For this review, take the finished solid that the model builds, in its own axes (mm). Face numbers are marked on the shaded views. A direction names the side the tool comes from. Coordinates: 2 decimals unless noted, no trailing zeros. Loops run counter-clockwise (first coordinate to the right, second up) from the corner with the lowest first, then second, coordinate; pieces in that order, holes last.
1. Mouldability with a two-part tool opening along X and no side actions: class the marked faces 1, 2, 3 and 4 as pulls with the +X half, pulls with the -X half, needs draft (parallel to the pull), parting line crosses it, or undercut.
2. Clearance check with flat-ended pins moving along their axes: P1, Ø3, axis at x = -59, z = 13, coming from the -Y side; P2, Ø1.5, axis at y = 9.5, z = 23, coming from the -X side; P3, Ø1, axis at x = -65.5, y = 8, coming from the -Z side. State where each tip first meets the part, or that it passes through.
3. Take a section at A-A, the plane x = 23.5. State the section outline as (y, z) points (3 decimals).
4. Machinability: for the marked faces 5 and 6, which of the approach directions +Z, -Z, +X, -X, +Y, -Y give a long, thin tool a straight path to every point of the face, cutting with its end or side? Answer none if there is none.
5. Take a section at B-B, the plane y = -9.5. State the section outline as (x, z) points.
6. To check wall thickness, follow probe 1 along Y at (x, z) = (-24.5, 4.5) (3 decimals); probe 2 along Z at (x, y) = (45.5, 2.5); probe 3 along X at (y, z) = (5, 9). State the ranges of each line that lie inside material, in increasing order.
```python
from build123d import *

# Parameters (mm, degrees)
F0_W        = 177.8
F0_H        = 44.45
F1_DEPTH    = 31.75
F2_W        = 2.032
F2_H        = 5.08
F2_H_2      = 2.957622528
F3_DEPTH    = 70.866
F4_T1_DEPTH = 472.3767319638
F5_R        = 10.16
F6_R        = 10.16
F7_R        = 8.5849434278
F8_W        = 78.1799629331
F8_H        = 27.9869418591
F9_DEPTH    = 12.7


# Not quite as in the source:
# - a fillet or chamfer that OpenCascade refuses, or shapes differently, is made with other operations: its cross-section is extruded or revolved along the edge and cut away or added


with BuildPart() as f1:
    # F0 (on Top) → F1 (new body)
    with BuildSketch(Plane.XY):
        Rectangle(F0_W, F0_H)
    extrude(amount=F1_DEPTH)

    # F2 (on Front) → F3 (cut, symmetric)
    with BuildSketch(Plane.XZ):
        with Locations((-65.8876, 0)):
            Rectangle(F2_W, F2_H)
        with Locations((45.8724, 1.061188736)):
            Rectangle(F2_W, F2_H_2)
    extrude(amount=F3_DEPTH, both=True, mode=Mode.SUBTRACT)

    # F4: fillet of radius 131.2269923964 on 1 edges, made by hand

    # F4_s2 → F4_t1 (cut)
    with BuildSketch(Plane.XZ.offset(-236.1883659819)):
        with BuildLine():
            ThreePointArc((-3.3146536072, 31.75), (-48.9570517069, 23.5567226134), (-88.9, 0))
            Line((-88.9, 0), (-88.9, 31.75))
            Line((-88.9, 31.75), (-3.3146536072, 31.75))
        make_face()
    extrude(amount=F4_T1_DEPTH, mode=Mode.SUBTRACT)

    # F5
    f5_edges = [f1.edges().sort_by_distance(p)[0] for p in [
        (-48.957052, -22.225, 23.556723),
    ]]
    fillet(f5_edges, radius=F5_R)

    # F6
    f6_edges = [f1.edges().sort_by_distance(p)[0] for p in [
        (42.792673, 22.225, 31.75),
        (-48.957052, 22.225, 23.556723),
    ]]
    fillet(f6_edges, radius=F6_R)

    # F7
    f7_edges = [f1.edges().sort_by_distance(p)[0] for p in [
        (88.9, 0, 31.75),
        (88.9, 22.225, 10.795),
        (88.9, -22.225, 10.795),
        (88.9, 19.249205, 28.774205),
        (88.9, -19.249205, 28.774205),
    ]]
    fillet(f7_edges, radius=F7_R)

    # F8 (on Top) → F9 (cut, symmetric)
    with BuildSketch(Plane.XY):
        Rectangle(F8_W, F8_H)
    extrude(amount=F9_DEPTH, both=True, mode=Mode.SUBTRACT)


solid = f1.part
```
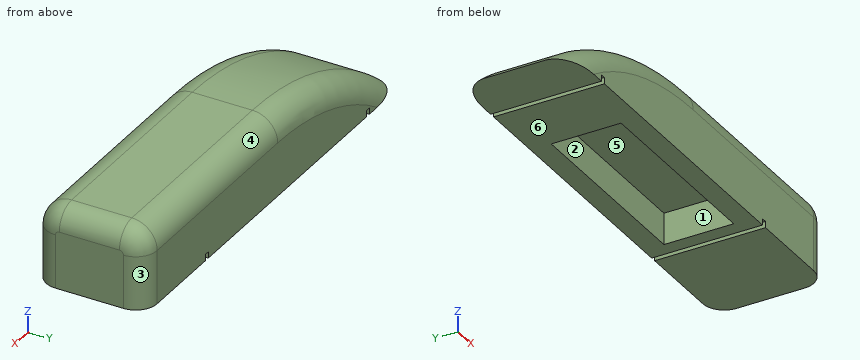
Results list:
1. face 1: undercut
1. face 2: undercut
1. face 3: pulls with the +X half
1. face 4: needs draft
2. P1: stops at y = -21.79
2. P2: stops at x = -52.34
2. P3: stops at z = 2.54
3. outline: (-22.225, 0) - (-13.993, 0) - (-13.993, 12.7) - (13.993, 12.7) - (13.993, 0) - (22.225, 0) - (22.225, 21.59) arc R10.16 ccw to (12.065, 31.75) - (-12.065, 31.75) arc R10.16 ccw to (-22.225, 21.59) - close
4. face 5: -Z
4. face 6: -Z, +X, -X, +Y, -Y
5. outline: (-88.9, 0) - (-66.9, 0) - (-66.9, 2.54) - (-64.87, 2.54) - (-64.87, 0) - (-39.09, 0) - (-39.09, 12.7) - (39.09, 12.7) - (39.09, 0) - (44.86, 0) - (44.86, 2.54) - (46.89, 2.54) - (46.89, 0) - (88.9, 0) - (88.9, 23.17) arc R8.58 ccw to (80.32, 31.75) - (-3.31, 31.75) arc R131.23 ccw to start
6. probe 1: y = -22.225 to -13.993, 13.993 to 22.225
6. probe 2: z = 2.54 to 31.75
6. probe 3: x = -77.16 to -39.09, 39.09 to 88.9
